```python
from build123d import *

# Parameters (mm, degrees)
BOSS_EXTRUDE1_DEPTH                                  = 110
FILLET1_R                                            = 25.4
FILLET2_R                                            = 10
SKETCH2_W                                            = 20
SKETCH2_H                                            = 23.04885876
CUT_EXTRUDE1_DEPTH                                   = 103.65
CBORE_FOR_1_4_BINDING_HEAD_MACHINE_SCREW_D           = 6.7564
CBORE_FOR_1_4_BINDING_HEAD_MACHINE_SCREW_CBORE_D     = 14.2875
CBORE_FOR_1_4_BINDING_HEAD_MACHINE_SCREW_CBORE_DEPTH = 4.191


with BuildPart() as part:
    # Sketch1 → Boss-Extrude1 (new body)
    with BuildSketch(Plane(origin=(0, 0, 0), x_dir=(0, 0, -1), z_dir=(1, 0, 0))):
        Polygon((0, 0), (20, 0), (20, 23.04885876), (60.747951032, 39.36618781), (101.495902064, 23.04885876), (101.495902064, 0), (121.495902064, 0), (121.495902064, 26.395679347), (110.865902064, 26.395679347), (60.747951032, 45.71618781), (10.63, 26.395679347), (0, 26.395679347), align=None)
    extrude(amount=BOSS_EXTRUDE1_DEPTH)

    # Fillet1
    # the kernel refuses this fillet: 25.4 mm, written as the material it takes off along each edge
    with BuildSketch(Plane(origin=(-51.660375289, 26.395679347, -121.495902064), x_dir=(0, -1, 0), z_dir=(1, 0, 0))) as fillet1_piece_1:
        with BuildLine():
            CenterArc((20.664150116, -25.4), FILLET1_R, 90, 54.444163321)
            Line((0, -10.63), (-0.413283002, -10.3346))
            ThreePointArc((-0.413283002, -10.3346), (-0.508, -5.315), (-0.508, 0))
            Line((-0.508, 0), (0, 0.508))
            Line((0, 0.508), (20.664150116, 0.508))
            Line((20.664150116, 0.508), (20.664150116, 0))
        make_face()
    extrude(amount=213.320750578, mode=Mode.SUBTRACT)
    with BuildSketch(Plane(origin=(-51.660375289, 26.395679347, 0), x_dir=(0, 0, -1), z_dir=(1, 0, 0))) as fillet1_piece_2:
        with BuildLine():
            CenterArc((25.4, -20.664150116), FILLET1_R, 125.555836679, 54.444163321)
            Line((0, -20.664150116), (-0.508, -20.664150116))
            Line((-0.508, -20.664150116), (-0.508, 0))
            Line((-0.508, 0), (0, 0.508))
            ThreePointArc((0, 0.508), (5.315, 0.508), (10.3346, 0.413283002))
            Line((10.3346, 0.413283002), (10.63, 0))
        make_face()
    extrude(amount=213.320750578, mode=Mode.SUBTRACT)
    with BuildSketch(Plane(origin=(-24.479298578, 45.71618781, -60.747951032), x_dir=(0, -0.35969863434758087, -0.9330685357724187), z_dir=(1, 0, 0))) as fillet1_piece_3:
        with BuildLine():
            CenterArc((FILLET1_R * 0.385500765011, -FILLET1_R), FILLET1_R, 90, 42.163378571)
            Line((-FILLET1_R * 0.285746191129, -FILLET1_R * 0.258766215103), (-FILLET1_R * 0.299171130252, -FILLET1_R * 0.243941539405))
            Line((-FILLET1_R * 0.299171130252, -FILLET1_R * 0.243941539405), (-FILLET1_R * 0.00771001530021, FILLET1_R * 0.02))
            Line((-FILLET1_R * 0.00771001530021, FILLET1_R * 0.02), (FILLET1_R * 0.385500765011, FILLET1_R * 0.02))
            Line((FILLET1_R * 0.385500765011, FILLET1_R * 0.02), (FILLET1_R * 0.385500765011, 0))
        make_face()
    extrude(amount=158.958597156, mode=Mode.SUBTRACT)

    # Fillet2
    fillet2_edges = [part.edges().sort_by_distance(p)[0] for p in [
        (55, 39.36618781, -60.747951032),
    ]]
    fillet(fillet2_edges, radius=FILLET2_R)

    # Sketch2 → Cut-Extrude1 (cut)
    with BuildSketch(Plane(origin=(110, 0, 0), x_dir=(0, 0, -1), z_dir=(1, 0, 0))):
        with Locations((10, 11.52442938)):
            Rectangle(SKETCH2_W, SKETCH2_H)
        with Locations((111.495902064, 11.52442938)):
            Rectangle(SKETCH2_W, SKETCH2_H)
    extrude(amount=-CUT_EXTRUDE1_DEPTH, mode=Mode.SUBTRACT)

    # CBORE for 1/4 Binding Head Machine Screw1 (through all)
    with Locations(Plane(origin=(6.35, 0, 0), x_dir=(0, 0, -1), z_dir=(1, 0, 0))):
        with Locations((9.21, 6.89), (112.285902064, 6.89)):
            CounterBoreHole(CBORE_FOR_1_4_BINDING_HEAD_MACHINE_SCREW_D / 2, CBORE_FOR_1_4_BINDING_HEAD_MACHINE_SCREW_CBORE_D / 2, CBORE_FOR_1_4_BINDING_HEAD_MACHINE_SCREW_CBORE_DEPTH)


solid = part.part
```
Read the model definition and answer for the solid it produces. Units are mm, in the model's axes. A direction names the side the tool comes from. Give positions to 0.01 mm unless a question says otherwise; leave off trailing zeros. Write each loop counter-clockwise with the first axis right and the second up, starting at its lowest first coordinate (ties: lowest second). Pieces come first, ordered by that corner, then holes. Notation, with made-up numbers: M -13,6.5 L 34,6.5 A8 ccw 34,16.5 Z; hole C 80.5,74 d11. An arc over 180 degrees is marked long. Put each result on its own line as item: value. Start each with the question number.
1. The part is cut by section B-B, the plane x = 60. Give the vertices of the cut face in (y, z).
2. Consider line 1 along Z through (x, y) = (3.45, 6.89); line 2 along Z through (x, y) = (1, 6); line 3 along X through (y, z) = (18, -102). Determine where each line is inside the solid, lowest interval first.
3. Which of the six approach directions +Z, -Z, +X, -X, +Y, -Y give full straight-line access (tool end or side, diameter ignored) to faces 4 (the cylindrical face through (4.284, 14.028, -9.497)), 5 (the flat face through (6.35, 14, -12)), 6 (the flat face through (3, 3, -121.496)), 7 (the flat face through (54.23, 30.567, -82.721)), 8 (the flat face through (3, 3, 0))?
4. For a pull along Y with two mould halves and no side action, classify faces 1 (the cylindrical face through (1.064, 7.905, -109.064)), 2 (the flat face through (54.23, 34.184, -90.662)), 3 (the flat face through (6.35, 14, -109)) as released by +Y, released by -Y, zero draft, split by the parting line, or undercut.
5. Each of these flat-tipped pins is pushed along its axis until it touches: pin 1 Ø10 at (y, z) = (20.5, -38) entering from +X; pin 2 Ø7 at (y, z) = (7, -7.5) entering from +X; pin 3 Ø1.9 at (x, y) = (2.5, 13.5) entering from +Z; pin 4 Ø6.5 at (x, z) = (51.5, -107.5) entering from -Y. Where does it stop, or does it pass through?
6. The part is cut by section D-D, the plane z = -91.5. Give the vertices of the cut face in (x, y).
7. The part is cut by section A-A, the plane z = -9.21. Give the vertices of the cut face in (x, y).
8. The part is cut by section C-C, the plane y = 12.5. Give the vertices of the cut face in (x, z), and give its area (3 significant figures).
Final values:
1. outline: M 23.05,-114.68 A25.4 ccw 26.4,-110.87 L 42.19,-69.88 A25.4 ccw 42.19,-51.61 L 26.4,-10.63 A25.4 ccw 23.05,-6.82 L 23.05,-20 L 37.88,-57.03 A10 cw 37.88,-64.47 L 23.05,-101.5 Z
2. line 1: z = -121.47 to -119.43, -105.14 to -101.5, -20 to -16.35, -2.07 to -0.03
2. line 2: z = -121.49 to -115.54, -109.03 to -101.5, -20 to -12.47, -5.95 to 0
2. line 3: x = 0 to 6.35
3. face 4: +X
3. face 5: +Z, -Z, +X, -Y
3. face 6: -Z, +X, -X, +Y, -Y
3. face 7: +X, -X, -Y
3. face 8: +Z, +X, -X, +Y, -Y
4. face 1: undercut
4. face 2: released by +Y
4. face 3: zero draft
5. pin 1: passes through
5. pin 2: stops at x = 2.16
5. pin 3: stops at z = -0.93
5. pin 4: stops at y = 23.05
6. outline: M 0,27.05 L 110,27.05 L 110,33.86 L 0,33.86 Z
7. outline: M 0,0 L 2.16,0 L 2.16,3.51 L 0,3.51 Z; M 0,10.27 L 2.16,10.27 L 2.16,14.03 L 6.35,14.03 L 6.35,23.05 L 110,23.05 L 110,25.3 L 0,25.3 Z
8. outline: M 0,-120.58 L 6.35,-120.58 L 6.35,-116.71 L 2.16,-116.71 L 2.16,-107.86 L 6.35,-107.86 L 6.35,-101.5 L 0,-101.5 Z; M 0,-20 L 6.35,-20 L 6.35,-13.63 L 2.16,-13.63 L 2.16,-4.79 L 6.35,-4.79 L 6.35,-0.92 L 0,-0.92 Z
8. area: 168 mm²
